Autodesk Inventor part; units mm, degrees
ref_plane "작업 평면1" through (-15, 25.5, -25) normal (-1, 0, 0) x (0, 0, 1)
ref_plane "YZ Plane" through (0, 0, 0) normal (1, 0, 0) x (0, 1, 0)
ref_plane "XZ Plane" through (0, 0, 0) normal (0, 1, 0) x (-1, 0, 0)
sketch "스케치1" plane through (0, 0, 0) normal (0, 0, 1) x (1, 0, 0)
  line L0 (-5, -35.5) -> (5, -35.5)
  line L1 (5, -35.5) -> (5, 35.5)
  line L2 (5, 35.5) -> (-5, 35.5)
  line L3 (-5, 35.5) -> (-5, -35.5)
  line L4 (-5, -35.5) -> (5, 35.5) construction
  line L5 (5, -35.5) -> (-5, 35.5) construction
  line L6 (-5, 35.5) -> (-35, 35.5)
  line L7 (-35, 35.5) -> (-35, 25.5)
  line L8 (-35, 25.5) -> (-5, 25.5)
  line L9 (-5, 25.5) -> (-5, 35.5)
  line L10 (0, 0) -> (-11.0402, 0)
  line L11 (-5, -35.5) -> (-35, -35.5)
  line L12 (-35, -35.5) -> (-35, -25.5)
  line L13 (-35, -25.5) -> (-5, -25.5)
  point P0 (-5, 25.5)
  point P1 (-5, -25.5)
  dimension "d0" = 71
  dimension "d1" = 10
  dimension "d2" = 10
  dimension "d3" = 30
extrude "돌출1" add sketch "스케치1" along normal mid plane 50
ref_plane "작업 평면1" through (-15, 25.5, -25) normal (-1, 0, 0) x (0, 0, 1)
sketch "스케치5" plane through (-5, -25.5, 25) normal (-1, 0, 0) x (0, 0, 1)
  line L0 (-50, 0) -> (0, 0)
  line L1 (0, 51) -> (0, 0)
  line L2 (-50, 51) -> (0, 51)
  line L3 (-50, 0) -> (-50, 51)
  line L4 (-8, 43) -> (-8, 8)
  line L5 (-8, 8) -> (-42, 8)
  line L6 (-42, 8) -> (-42, 43)
  line L7 (-42, 43) -> (-8, 43)
  line L8 (-42, 43) -> (-8, 8) construction
  line L9 (-36.4234, 43) -> (-8, 13.7406)
  line L10 (-42, 37.2594) -> (-13.5766, 8)
  line L11 (-25, 25.5) -> (-25, 37.0316)
  line L12 (-8, 43) -> (-42, 8) construction
  line L13 (-13.5766, 43) -> (-42, 13.7406)
  line L14 (-8, 37.2594) -> (-36.4234, 8)
  point P0 (-42, 13.7406)
  point P1 (-30.5766, 25.5)
  point P2 (-8, 37.2594)
  point P3 (-19.4234, 25.5)
  point P4 (-25, 19.7594)
  point P5 (-36.4234, 8)
  point P6 (-25, 31.2406)
  dimension "d24" = 8
  dimension "d25" = 4
  dimension "d26" = 4
extrude "돌출5" cut sketch "스케치5" against normal blind 10 contours L4 L9 L14 | L13 L9 L7 | L10 L5 L14 | L13 L6 L10
fillet "모깎기1" radius 2 2 edges at (-5, 25.5, 0) (-5, -25.5, 0)
sketch "스케치6" plane through (-35, -35.5, 25) normal (0, -1, 0) x (1, 0, 0)
  circle A0 centre (12, -25) radius 5
  line L0 (0, -50) -> (0, 0)
  point P0 (35, -25)
  point P1 (0, -25)
  dimension "d30" = 10
  dimension "d31" = 12
extrude "돌출6" cut sketch "스케치6" against normal up to surface (10 mm away)
chamfer "모따기1" distance 15 angle 45 2 edges at (-35, -30.5, 25) (-35, -30.5, -25)
sketch "스케치7" plane through (-7, -25.5, 25) normal (0, 1, 0) x (1, 0, 0)
  circle A0 centre (-16, 25) radius 5
  line L0 (-16, 35.0459) -> (-7.3, 30.0229)
  line L1 (-7.3, 30.0229) -> (-7.3, 19.9771)
  line L2 (-7.3, 19.9771) -> (-16, 14.9541)
  line L3 (-16, 14.9541) -> (-24.7, 19.9771)
  line L4 (-24.7, 19.9771) -> (-24.7, 30.0229)
  line L5 (-24.7, 30.0229) -> (-16, 35.0459)
  point P0 (7, 25)
  dimension "d37" = 17.4
extrude "돌출7" cut sketch "스케치7" against normal blind 6 contours A0 | L0 L1 L2 L3 L4 L5
sketch "스케치14" plane through (-35, 25.5, -25) normal (0, -1, 0) x (1, 0, 0)
  circle A0 centre (5, 5) radius 1.75
  circle A1 centre (5, 5) radius 3
  line L0 (0, 0) -> (40, 0)
  line L1 (0, 0) -> (0, 50)
  circle A2 centre (15, 5) radius 1.75
  circle A3 centre (15, 5) radius 3
  circle A4 centre (25, 5) radius 1.75
  circle A5 centre (25, 5) radius 3
  point P0 (35, 25)
  dimension "d74" = 3.5
  dimension "d75" = 6
  dimension "d76" = 5
  dimension "d77" = 5
  dimension "d80" = 10
extrude "돌출12" cut sketch "스케치14" against normal blind 10 contours A0 | A2 | A4
extrude "돌출13" cut sketch "스케치14" against normal blind 2.5 contours A1 | A3 | A4 | A5
sketch "스케치15" plane through (-35, 35.5, 25) normal (0, 1, 0) x (1, 0, 0)
  circle A0 centre (20, 8) radius 1.75
  line L0 (40, 0) -> (0, 0)
  line L1 (40, 50) -> (40, 0)
  circle A1 centre (20, 20) radius 1.75
  circle A2 centre (20, 32) radius 1.75
  point P0 (35, 25)
  point P1 (20, 0)
  dimension "d89" = 3.5
  dimension "d90" = 8
  dimension "d93" = 12
extrude "돌출14" cut sketch "스케치15" against normal up to surface (10 mm away)
chamfer "모따기3" distance 10 angle 45 1 edges at (-35, 30.5, 25)
chamfer "모따기4" distance 5 angle 45 1 edges at (5, -35.5, 0)
sketch "스케치16" plane through (-35, 25.5, -25) normal (0, -1, 0) x (1, 0, 0)
  circle A0 centre (20, 18) radius 1.75
  circle A1 centre (20, 18) radius 3
  circle A2 centre (20, 30) radius 1.75
  circle A3 centre (20, 30) radius 3
  circle A4 centre (20, 42) radius 1.75
  circle A5 centre (20, 42) radius 3
  point P0 (35, 25)
  dimension "d106" = 6
  dimension "d107" = 6
  dimension "d108" = 6
extrude "돌출15" cut sketch "스케치16" against normal blind 2.5 contours A0 | A1 | A2 | A3 | A4 | A5
properties part number "전체 형상"
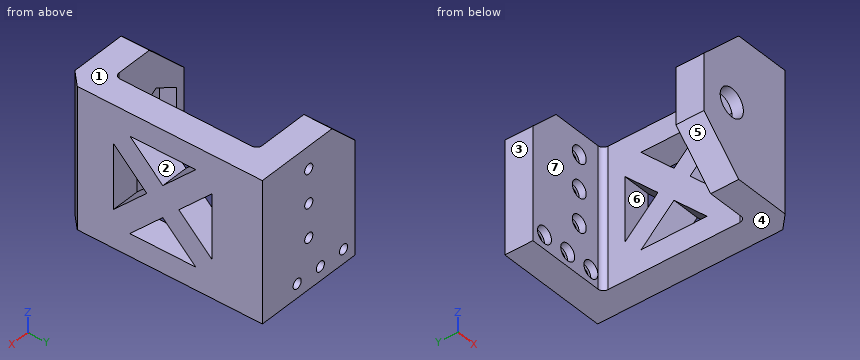
Input: part model. Units: mm. Frame: model coordinates. Face numbers are marked on the shaded views. A direction names the side the tool comes from. Coordinates: 2 decimals unless noted, no trailing zeros. Loops run counter-clockwise (first coordinate to the right, second up) from the corner with the lowest first, then second, coordinate; pieces in that order, holes last.
Q1. Set-up query: the marked faces 5, 6 and 7. Return all of +Z, -Z, +X, -X, +Y, -Y with unobstructed straight access to the full face (end or side cutting, diameter ignored); none if empty.
Q2. Cut plane D-D (z = -13). Output: boundary loops of the cut face in (x, y), then the cut area to 3 significant figures.
Q3. Cut plane A-A (x = -10). Output: boundary loops of the cut face in (y, z), then the cut area to 3 significant figures.
Q4. Draft query along Z for the marked faces 1, 2, 3 and 4. Return one class per face: +Z half, -Z half, draft (parallel to the pull), parting line (faces both ways), or undercut.
Q5. Cut plane B-B (x = 3). Output: boundary loops of the cut face in (y, z).
Q6. Cut plane C-C (y = -29.5). Output: boundary loops of the cut face in (x, z).
Q7. Material intervals for line 1 (Z direction, x = -20, y = 34.25); line 2 (Y direction, x = 3, z = 8.5); line 3 (Z direction, x = -15, y = 30), sorted ascending.
Q8. Contact query for flat-ended pins moving along their axis: pin 1 (1.5 mm diameter, centred on y = 21, z = 13.5, fed in from -X); pin 2 (1.5 mm diameter, centred on y = 24.5, z = 17, fed in from -X); pin 3 (12 mm diameter, centred on y = -25, z = 19.5, fed in from -X); pin 4 (1.5 mm diameter, centred on y = 1.5, z = 14.5, fed in from +X). Output: stop coordinate, or through.
Working result:
1. face 5: -Z, -X, -Y
1. face 6: +X, -X
1. face 7: +Z, -Z, -X
2. outline: (-35, 25.5) - (-7, 25.5) arc R2 cw to (-5, 23.5) - (-5, 7.64) - (5, 7.64) - (5, 35.5) - (-35, 35.5) - close; (-32, -35.5) - (0, -35.5) - (5, -30.5) - (5, -7.64) - (-5, -7.64) - (-5, -23.5) arc R2 cw to (-7, -25.5) - (-32, -25.5) - close
2. area: 1,120 mm2
3. outline: (-35.5, -25) - (-25.5, -25) - (-25.5, 25) - (-35.5, 25) - close; (25.5, -25) - (35.5, -25) - (35.5, -21.75) - (28, -21.75) - (28, -23) - (25.5, -23) - close; (25.5, -17) - (28, -17) - (28, -18.25) - (35.5, -18.25) - (35.5, 25) - (25.5, 25) - close
3. area: 959 mm2
4. face 1: +Z half
4. face 2: undercut
4. face 3: draft
4. face 4: -Z half
5. outline: (-32.5, -25) - (35.5, -25) - (35.5, 25) - (-32.5, 25) - close; hole (-17.5, -11.42) - (-5.74, 0) - (-17.5, 11.42) - close; hole (-11.76, -17) - (11.76, -17) - (0, -5.58) - close; hole (-11.76, 17) - (0, 5.58) - (11.76, 17) - close; hole (5.74, 0) - (17.5, -11.42) - (17.5, 11.42) - close
6. outline: (-35, -10) - (-20, -25) - (5, -25) - (5, 25) - (-20, 25) - (-35, 10) - close; hole (-31.7, -5.02) - (-23, -10.05) - (-14.3, -5.02) - (-14.3, 5.02) - (-23, 10.05) - (-31.7, 5.02) - close
7. line 1: z = -25 to -21.75, -18.25 to 25
7. line 2: y = -32.5 to -17.5, -14.49 to -3.01, 3.01 to 14.49, 17.5 to 35.5
7. line 3: z = -25 to -8.75, -5.25 to 3.25, 6.75 to 15.25, 18.75 to 25
8. pin 1: stops at x = -5
8. pin 2: stops at x = -6.03
8. pin 3: stops at x = -31.48
8. pin 4: passes through
